The figure shows three views and two pictorial views of one solid part (mm, origin at its lowest corner). Answer the questions. A direction names the side the tool comes from. Round coordinates to 2 decimals unless told otherwise and drop trailing zeros. Write each loop counter-clockwise with the first axis right and the second up, starting at its lowest first coordinate (ties: lowest second). Pieces come first, ordered by that corner, then holes.
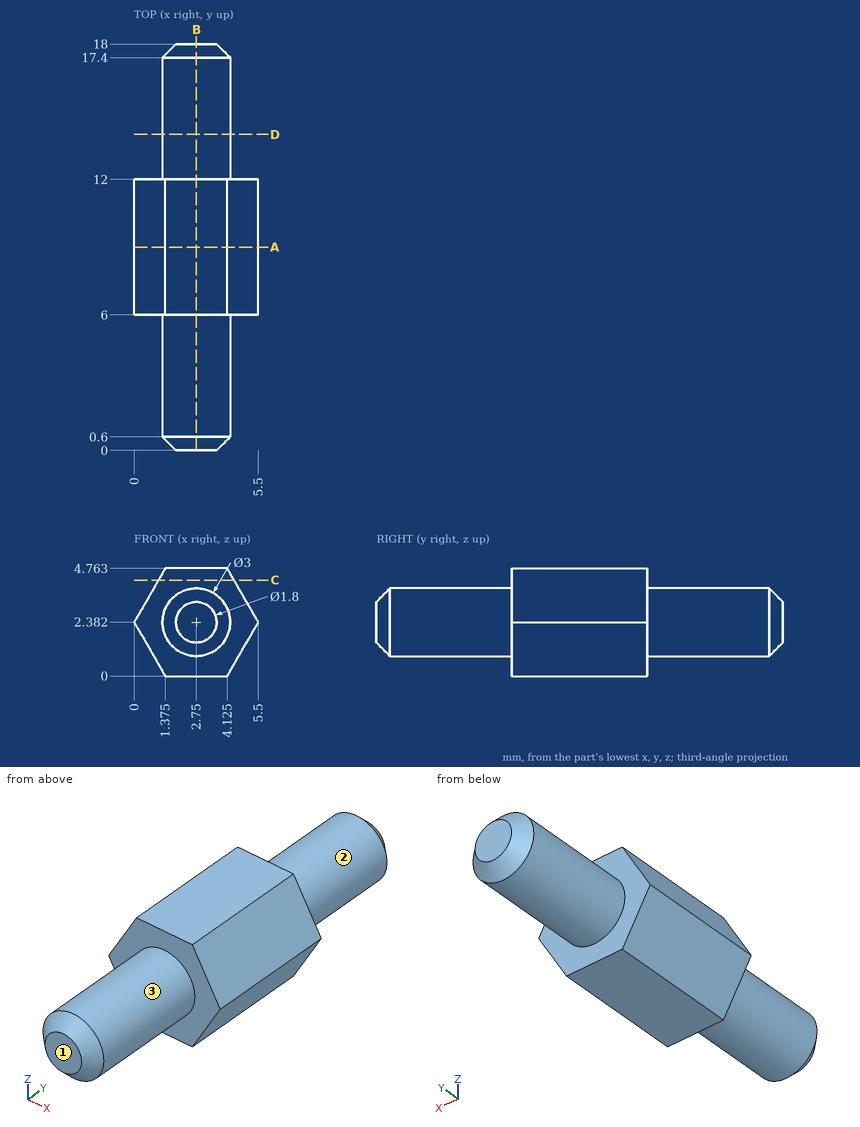
Q1. Section C-C (z = 4.25) is taken. Determine the outline of the cut face in (x, y).
Verdict:
outline: (1.08, 6) - (4.42, 6) - (4.42, 12) - (1.08, 12) - close
Q2. Section A-A (y = 9) is taken. Determine the outline of the cut face in (x, z) (1 decimal).
Verdict:
outline: (0, 2.4) - (1.4, 0) - (4.1, 0) - (5.5, 2.4) - (4.1, 4.8) - (1.4, 4.8) - close
Q3. Which of the six approach directions +Z, -Z, +X, -X, +Y, -Y give full straight-line access (tool end or side, diameter ignored) to the marked faces 1, 2 and 3?
Verdict:
face 1: +Z, -Z, +X, -X, -Y
face 2: +Y
face 3: -Y
Q4. Straight lines are drawn through the part: probe 1 along Y at (x, z) = (0.4, 2.1); probe 2 along Z at (x, y) = (3.8, 14) (1 decimal); probe 3 along X at (y, z) = (7.5, 1.9). For each, find the intervals that lie inside material, in ascending order.
Verdict:
probe 1: y = 6 to 12
probe 2: z = 1.3 to 3.5
probe 3: x = 0.28 to 5.22
Q5. Section D-D (y = 14) is taken. Determine the outline of the cut face in (x, z).
Verdict:
outline: circle Ø3 at (2.75, 2.38)
Q6. Section B-B (x = 2.75) is taken. Determine the outline of the cut face in (y, z).
Verdict:
outline: (0, 1.48) - (0.6, 0.88) - (6, 0.88) - (6, 0) - (12, 0) - (12, 0.88) - (17.4, 0.88) - (18, 1.48) - (18, 3.28) - (17.4, 3.88) - (12, 3.88) - (12, 4.76) - (6, 4.76) - (6, 3.88) - (0.6, 3.88) - (0, 3.28) - close
